Could you check a few things on this model? Use its own coordinates, in mm. Face numbers are marked on the shaded views. A direction names the side the tool comes from. Give positions to 0.01 mm unless a question says otherwise; leave off trailing zeros. Write each loop counter-clockwise with the first axis right and the second up, starting at its lowest first coordinate (ties: lowest second). Pieces come first, ordered by that corner, then holes. Notation, with made-up numbers: (50.5, 35) - (83.5, 35) arc R27 cw to (83.5, 71) - close; hole circle Ø7 at (59, 73). An arc over 180 degrees is marked (long way). Write item = value, one per line.
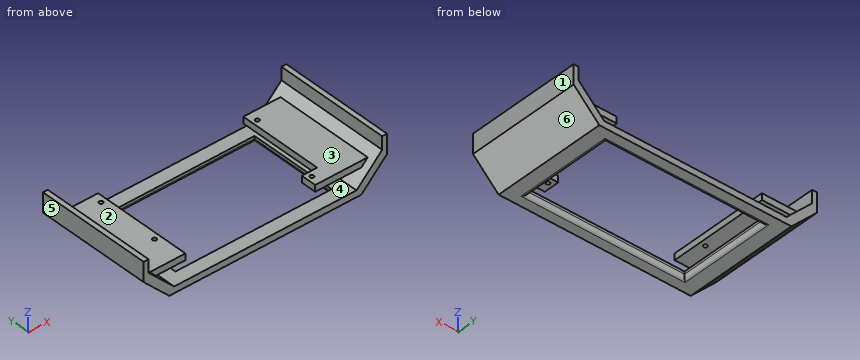
from build123d import *

# Parameters (mm, degrees)
SKETCH1_W           = 190
SKETCH1_H           = 90
SKETCH1_W_2         = 122
SKETCH1_H_2         = 69
BOSS_EXTRUDE1_DEPTH = 5
SKETCH2_W           = 3.8
SKETCH2_H           = 90
BOSS_EXTRUDE2_DEPTH = 30
SKETCH3_W           = 34
SKETCH3_H           = 5
SKETCH3_W_2         = 47
BOSS_EXTRUDE3_DEPTH = 90
SKETCH4_W           = 182.4
SKETCH4_H           = 6
CUT_EXTRUDE1_DEPTH  = 5
SKETCH5_R           = 1.5
CUT_EXTRUDE2_DEPTH  = 5
SKETCH6_W           = 12
SKETCH6_H           = 66
CUT_EXTRUDE3_DEPTH  = 5
FILLET3_R           = 3
CHAMFER6_SIZE       = 20


with BuildPart() as part:
    # Sketch1 → Boss-Extrude1 (new body)
    with BuildSketch(Plane.XY):
        Rectangle(SKETCH1_W, SKETCH1_H)
        Rectangle(SKETCH1_W_2, SKETCH1_H_2, mode=Mode.SUBTRACT)
    extrude(amount=BOSS_EXTRUDE1_DEPTH)

    # Sketch2 → Boss-Extrude2 (add)
    with BuildSketch(Plane.XY.offset(5)):
        with Locations((-93.1, 0)):
            Rectangle(SKETCH2_W, SKETCH2_H)
        with Locations((93.1, 0)):
            Rectangle(SKETCH2_W, SKETCH2_H)
    extrude(amount=BOSS_EXTRUDE2_DEPTH)

    # Sketch3 → Boss-Extrude3 (add)
    with BuildSketch(Plane(origin=(0, 45, 0), x_dir=(1, 0, 0), z_dir=(0, 1, 0))):
        with Locations((-74.2, -16.5)):
            Rectangle(SKETCH3_W, SKETCH3_H)
        with Locations((67.7, -16.5)):
            Rectangle(SKETCH3_W_2, SKETCH3_H)
    extrude(amount=-BOSS_EXTRUDE3_DEPTH)

    # Sketch4 → Cut-Extrude1 (cut)
    with BuildSketch(Plane.XY.offset(19)):
        with Locations((0, 42)):
            Rectangle(SKETCH4_W, SKETCH4_H)
        with Locations((0, -42)):
            Rectangle(SKETCH4_W, SKETCH4_H)
    extrude(amount=-CUT_EXTRUDE1_DEPTH, mode=Mode.SUBTRACT)

    # Sketch5 → Cut-Extrude2 (cut)
    with BuildSketch(Plane.XY.offset(19)):
        with Locations((-61.75, 31.13)):
            Circle(SKETCH5_R)
        with Locations((-61.75, -16.61)):
            Circle(SKETCH5_R)
        with Locations((60.23, 31.13)):
            Circle(SKETCH5_R)
        with Locations((48.25, -31.38)):
            Circle(SKETCH5_R)
    extrude(amount=-CUT_EXTRUDE2_DEPTH, mode=Mode.SUBTRACT)

    # Sketch6 → Cut-Extrude3 (cut)
    with BuildSketch(Plane.XY.offset(19)):
        with Locations((50.2, 6)):
            Rectangle(SKETCH6_W, SKETCH6_H)
    extrude(amount=-CUT_EXTRUDE3_DEPTH, mode=Mode.SUBTRACT)

    # Fillet3
    fillet3_edges = [part.edges().sort_by_distance(p)[0] for p in [
        (61, 0, 0),
        (0, 34.5, 0),
        (-61, 0, 0),
        (0, -34.5, 0),
    ]]
    fillet(fillet3_edges, radius=FILLET3_R)

    # Chamfer6
    # the kernel refuses this chamfer: 20 mm, written as the material it adds along each edge
    with BuildSketch(Plane(origin=(-91.2, 45, 5), x_dir=(-0.027495876610586317, 0, 0.9996219169112968), z_dir=(0, -1, 0))) as chamfer6_piece_1:
        Polygon((CHAMFER6_SIZE * 0.999621916911, -CHAMFER6_SIZE * 0.0274958766106), (-CHAMFER6_SIZE * 0.0274958766106, -CHAMFER6_SIZE * 0.999621916911), (0, 0), align=None)
    extrude(amount=90)
    with BuildSketch(Plane(origin=(91.2, -45, 5), x_dir=(-0.9996219169112968, 0, -0.02749587661058636), z_dir=(0, 1, 0))) as chamfer6_piece_2:
        Polygon((CHAMFER6_SIZE * 0.999621916911, CHAMFER6_SIZE * 0.0274958766106), (-CHAMFER6_SIZE * 0.0274958766106, CHAMFER6_SIZE * 0.999621916911), (0, 0), align=None)
    extrude(amount=90)
    # the kernel refuses this chamfer: 20 mm, written as the material it takes off along each edge
    with BuildSketch(Plane(origin=(-95, -96.433659759, 0), x_dir=(0.9996219169112968, 0, -0.027495876610586372), z_dir=(0, 1, 0)), Plane(origin=(95, 96.433659759, 0), x_dir=(-0.9996219169112968, 0, -0.027495876610586372), z_dir=(0, -1, 0))) as chamfer6_2_piece_1:
        Polygon((CHAMFER6_SIZE * 0.999621916911, -CHAMFER6_SIZE * 0.0274958766106), (-CHAMFER6_SIZE * 0.0274958766106, -CHAMFER6_SIZE * 0.999621916911), (0, 0), align=None)
    extrude(amount=192.867319519, mode=Mode.SUBTRACT)


solid = part.part
1. Thinking about a two-plate mould opening in X: for the marked faces 3, 4, 5 and 6, which applies, pulls with the +X half, pulls with the -X half, needs draft (parallel to the pull), parting line crosses it, or undercut?
Filled sheet:
face_3 = undercut
face_4 = undercut
face_5 = pulls with the -X half
face_6 = pulls with the +X half
2. If we section it at A-A, the plane y = -9.5: Please give me the cut outline in (x, z), and give its area (3 significant figures).
Filled sheet:
outline = (-95, 20) - (-75, 0) - (-64, 0) arc R3 ccw to (-61, 3) - (-61, 5) - (-71.2, 5) - (-80.2, 14) - (-57.2, 14) - (-57.2, 19) - (-85.2, 19) - (-91.2, 25) - (-91.2, 35) - (-95, 35) - close; (56.2, 14) - (80.2, 14) - (71.2, 5) - (61, 5) - (61, 3) arc R3 ccw to (64, 0) - (75, 0) - (95, 20) - (95, 35) - (91.2, 35) - (91.2, 25) - (85.2, 19) - (56.2, 19) - close
area = 824 mm2
3. If we section it at C-C, the plane z = 31.5: Please give me the cut outline in (x, y), and give its area (3 significant figures).
Filled sheet:
outline = (-95, -45) - (-91.2, -45) - (-91.2, 45) - (-95, 45) - close; (91.2, -45) - (95, -45) - (95, 45) - (91.2, 45) - close
area = 684 mm2
4. If we section it at B-B, the plane x = -53: Please give me the cut outline in (y, z).
Filled sheet:
outline = (-45, 0) - (-37.5, 0) arc R3 ccw to (-34.5, 3) - (-34.5, 5) - (-45, 5) - close; (34.5, 3) arc R3 ccw to (37.5, 0) - (45, 0) - (45, 5) - (34.5, 5) - close
5. Which directions (+Z, -Z, +X, -X, +Y, -Y) give clear straight access to the entire face, cutting with the end or side of a thin tool? Please do the marked faces 1 and 2.
Filled sheet:
face_1 = +Z, -Z, +X, +Y, -Y
face_2 = +Z, +Y, -Y
6. For pin 1 (1.8 mm diameter, centred on x = -61.75, y = -16.61, fed in from +Z); pin 2 (5.5 mm diameter, centred on y = 14.5, z = 15.5, fed in from +X); pin 3 (2 mm diameter, centred on x = -56.5, y = 35, fed in from -Z); pin 4 (2.5 mm diameter, centred on x = 48.25, y = -31.38, fed in from +Z), each with a flat end and sliding along its axis, tell me the tip position at first contact or that it passes through.
Filled sheet:
pin_1 = 5
pin_2 = 93.25
pin_3 = 0.4
pin_4 = through
7. I need wall thicknesses on line 1 (X direction, y = 5, z = 34); line 2 (Y direction, x = 60, z = 17); line 3 (Y direction, x = 31, z = 4). Which ranges of each line are inside material? Lowest first, please.
Filled sheet:
line_1 = -95 to -91.2, 91.2 to 95
line_2 = -39 to 29.65, 32.61 to 39
line_3 = -45 to -34.5, 34.5 to 45
